The listing builds one solid part. Answer for the finished solid, in the listing's coordinates (mm). Face numbers are marked on the shaded views. Coordinates: 2 decimals unless noted, no trailing zeros. Order: outer loops, then holes, each group sorted by start corner. A loop starts at its lowest first (then second) coordinate and runs counter-clockwise, first axis right, second up. Notation, with made-up numbers: (44, -22) -> (56, -22) arc R30 cw to (56, 7) -> close; hole circle Ø2 at (-7, 50). An arc over 180 degrees is marked (long way). One line per question, with ' | ' between items.
from build123d import *

# Parameters (mm, degrees)
F0_R     = 8
F1_DEPTH = 41.4
F2_R     = 4.05
F2_W     = 5.5
F2_H     = 2.5
F3_DEPTH = 12.5
F4_R     = 1.5
F5_DEPTH = 16
F6_R     = 1.35
F7_DEPTH = 20
F8_R     = 2


with BuildPart() as f1:
    # F0 (on Top) → F1 (new body)
    with BuildSketch(Plane.XY):
        Circle(F0_R)
    extrude(amount=F1_DEPTH)

    # F2 (on Front) → F3 (cut, symmetric)
    with BuildSketch(Plane.XZ):
        with Locations((0, 27.4)):
            Circle(F2_R)
        with Locations((0, 34.7)):
            Rectangle(F2_W, F2_H)
    extrude(amount=F3_DEPTH, both=True, mode=Mode.SUBTRACT)

    # F4 (on face) → F5 (cut)
    with BuildSketch(Plane.XY.offset(41.4)):
        Circle(F4_R)
    extrude(amount=-F5_DEPTH, mode=Mode.SUBTRACT)

    # F6 (on face) → F7 (cut)
    with BuildSketch(Plane(origin=(0, 0, 0), x_dir=(1, 0, 0), z_dir=(0, 0, -1))):
        Circle(F6_R)
    extrude(amount=-F7_DEPTH, mode=Mode.SUBTRACT)

    # F8
    f8_edges = [f1.edges().sort_by_distance(p)[0] for p in [
        (-8, 0, 41.4),
    ]]
    fillet(f8_edges, radius=F8_R)


solid = f1.part
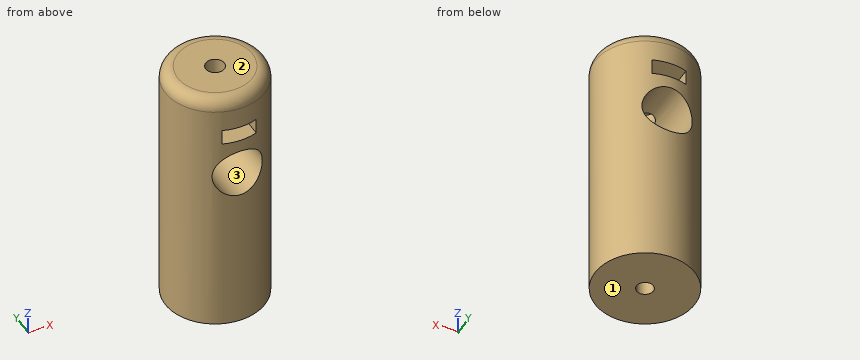
Item 1: Find the intervals of material crossed by L1, parallel to Y at x = 0, z = 5; L2, parallel to Y at x = 0, z = 32.75; L3, parallel to Z at x = 2, y = -0.5, in increasing order.
Computed values:
L1: y = -8 to -1.35, 1.35 to 8 | L2: y = -8 to -1.5, 1.5 to 8 | L3: z = 0 to 23.88, 30.92 to 33.45, 35.95 to 41.4
Item 2: Section A-A, the plane x = 0 is taken. Give the vertices of the cut face in (y, z), plus the area to 3 significant figures.
Computed values:
outline: (-8, 0) -> (-1.35, 0) -> (-1.35, 20) -> (1.35, 20) -> (1.35, 0) -> (8, 0) -> (8, 23.35) -> (-8, 23.35) -> close; (-8, 31.45) -> (-1.5, 31.45) -> (-1.5, 33.45) -> (-8, 33.45) -> close; (-8, 35.95) -> (-1.5, 35.95) -> (-1.5, 41.4) -> (-6, 41.4) arc R2 ccw to (-8, 39.4) -> close; (1.5, 31.45) -> (8, 31.45) -> (8, 33.45) -> (1.5, 33.45) -> close; (1.5, 35.95) -> (8, 35.95) -> (8, 39.4) arc R2 ccw to (6, 41.4) -> (1.5, 41.4) -> close | area: 415 mm^2
Item 3: Section B-B, the plane y = 0 is taken. Give the vertices of the cut face in (x, z).
Computed values:
outline: (-8, 0) -> (-1.35, 0) -> (-1.35, 20) -> (1.35, 20) -> (1.35, 0) -> (8, 0) -> (8, 39.4) arc R2 ccw to (6, 41.4) -> (1.5, 41.4) -> (1.5, 35.95) -> (2.75, 35.95) -> (2.75, 33.45) -> (1.5, 33.45) -> (1.5, 31.16) arc R4.05 cw (long way) to (-1.5, 31.16) -> (-1.5, 33.45) -> (-2.75, 33.45) -> (-2.75, 35.95) -> (-1.5, 35.95) -> (-1.5, 41.4) -> (-6, 41.4) arc R2 ccw to (-8, 39.4) -> close
Item 4: Each of these flat-tipped pins is pushed along its axis until it touches: pin 1 Ø2.5 at (x, y) = (0, 0) entering from +Z; pin 2 Ø6 at (y, z) = (-5.5, 22) entering from +X; pin 3 Ø3 at (y, z) = (-3, 12) entering from -X; pin 4 Ø7.5 at (x, z) = (0, 27.4) entering from +Y. Where does it stop, or does it pass through?
Computed values:
pin 1: stops at z = 23.55 | pin 2: stops at x = 7.6 | pin 3: stops at x = -7.86 | pin 4: passes through
Item 5: Section C-C, the plane z = 18 is taken. Give the vertices of the cut face in (x, y), plus the area to 3 significant figures.
Computed values:
outline: circle Ø16 at (0, 0); hole circle Ø2.7 at (0, 0) | area: 195 mm^2
Item 6: Determine the mould class of the marked faces 1, 2 and 3 for opening direction Z: pulls with the +Z half, pulls with the -Z half, needs draft (parallel to the pull), parting line crosses it, or undercut.
Computed values:
face 1: pulls with the -Z half | face 2: pulls with the +Z half | face 3: undercut
Item 7: Section D-D, the plane z = 27.4 is taken. Give the vertices of the cut face in (x, y).
Computed values:
outline: (-4.05, -6.9) -> (-4.05, 6.9) arc R8 ccw to start; (4.05, -6.9) arc R8 ccw to (4.05, 6.9) -> close
